```python
from build123d import *

# Parameters (mm, degrees)
ESQUISSE3_R             = 1
ENL_V_MAT_EXTRU_1_DEPTH = 5


with BuildPart() as part:
    # Esquisse1 → Révolution1 (revolve)
    with BuildSketch(Plane.XY, mode=Mode.PRIVATE) as r_volution1_sk:
        Polygon((0, 0), (14, 0), (14, 17), (14, 45), (13.5, 45.5), (13.5, 46.5), (13, 47), (11.5, 47), (11.5, 81), (7.5, 81), (7.5, 82), (4, 82), (4, 83), (3, 83), (3, 93), (0, 93), align=None)
    revolve(r_volution1_sk.sketch.rotate(Axis((0, 0, 0), (0, 1, 0)), 90), axis=Axis((0, 0, 0), (0, 1, 0)))

    # Esquisse3 → Enlèv. mat.-Extru.1 (cut)
    with BuildSketch(Plane(origin=(0, 81, 0), x_dir=(1, 0, 0), z_dir=(0, 1, 0))):
        with Locations(Location((9.5, 0, 0), (0, 0, 270))):
            Circle(ESQUISSE3_R)
        with Locations(Location((-4.75, -8.227241336, 0), (0, 0, 270))):
            Circle(ESQUISSE3_R)
        with Locations(Location((-4.75, 8.227241336, 0), (0, 0, 270))):
            Circle(ESQUISSE3_R)
    extrude(amount=-ENL_V_MAT_EXTRU_1_DEPTH, mode=Mode.SUBTRACT)


solid = part.part
```
The model under review builds one solid part; all positions refer to its coordinate system, in mm. A direction names the side the tool comes from. Coordinates: 2 decimals unless noted, no trailing zeros. Write each loop counter-clockwise with the first axis right and the second up, starting at its lowest first coordinate (ties: lowest second). Pieces come first, ordered by that corner, then holes. Notation, with made-up numbers: (-23.75, 17) - (34.25, 17) arc R14 ccw to (34.25, 42) - close; hole circle Ø3 at (-32.75, 87). An arc over 180 degrees is marked (long way). Write item = value, one per line.
(1) Mouldability with a two-part tool opening along Z and no side actions: class faces 1 (the face through (10.49, 78.54, -0.13)), 2 (the face through (-11.4, 64.2, 1.5)), 3 (the face through (0, 93, 0)), 4 (the face through (-5, 76, -8)) as pulls with the +Z half, pulls with the -Z half, needs draft (parallel to the pull), parting line crosses it, or undercut.
Result sheet:
face_1 = undercut
face_2 = parting line crosses it
face_3 = needs draft
face_4 = undercut
(2) Consider section B-B, the plane y = 77. Give the boundary of the cut face in (x, z).
Result sheet:
outline = circle Ø23 at (0, 0); hole circle Ø2 at (-4.75, -8.23); hole circle Ø2 at (-4.75, 8.23); hole circle Ø2 at (9.5, 0)
(3) Consider section C-C, the plane x = 0. Give the boundary of the cut face in (y, z), then the cut area to 3 significant figures.
Result sheet:
outline = (0, -14) - (45, -14) - (45.5, -13.5) - (46.5, -13.5) - (47, -13) - (47, -11.5) - (81, -11.5) - (81, -7.5) - (82, -7.5) - (82, -4) - (83, -4) - (83, -3) - (93, -3) - (93, 3) - (83, 3) - (83, 4) - (82, 4) - (82, 7.5) - (81, 7.5) - (81, 11.5) - (47, 11.5) - (47, 13) - (46.5, 13.5) - (45.5, 13.5) - (45, 14) - (0, 14) - close
area = 2,180 mm^2
(4) Machinability: for faces 5 (the face through (-5, 76, 8)), 6 (the face through (0, 0, 0)), which of the approach directions +Z, -Z, +X, -X, +Y, -Y give a long, thin tool a straight path to every point of the face, cutting with its end or side? Answer none if there is none.
Result sheet:
face_5 = +Y
face_6 = +Z, -Z, +X, -X, -Y
(5) For line 1 (X direction, y = 79.3, z = 0); line 2 (X direction, y = 35.5, z = 8); line 3 (X direction, y = 25.5, z = 3.75), list the stretches that pass through material, from the lowest coordinate up. Write a range as [from, to].
Result sheet:
line_1 = [-11.5, 8.5], [10.5, 11.5]
line_2 = [-11.49, 11.49]
line_3 = [-13.49, 13.49]
(6) Consider section D-D, the plane y = 28.5. Give the boundary of the cut face in (x, z), then the cut area to 3 significant figures.
Result sheet:
outline = circle Ø28 at (0, 0)
area = 616 mm^2
(7) For P1, Ø4, axis at y = 39.5, z = 5, coming from the -X side; P2, Ø3, axis at x = -9, y = 40, coming from the +Z side; P3, Ø4, axis at x = -0.5, y = 41.5, coming from the +Z side; P4, Ø4, axis at x = -1.5, y = 47.5, coming from the -Z side, all flat-tipped, find the tip position at first contact; note any pin that passes through.
Result sheet:
P1 = -13.67
P2 = 11.82
P3 = 14
P4 = -13.5
